Design review of the part built by this model. Coordinates are the model's own, in mm. A direction names the side the tool comes from. Give positions to 0.01 mm unless a question says otherwise; leave off trailing zeros. Loops run counter-clockwise (first coordinate to the right, second up) from the corner with the lowest first, then second, coordinate; pieces in that order, holes last. Notation, with made-up numbers: (11.25, 3) -> (31.25, 3) arc R25 ccw to (31.25, 30) -> close; hole circle Ø1 at (-8, 18.25). An arc over 180 degrees is marked (long way). Answer in a Markdown table with one row per item. Add a question column.
(1) Consider section D-D on y = 18. Write out the cut boundary in (x, z).
(2) For faces 1 (the cylindrical face through (17.923, -1.509, 1.726)), 2 (the flat face through (-48, 8.388, 2)), 3 (the flat face through (-38.16, -9.16, 1.73)), list the 3-axis set-ups (+Z, -Z, +X, -X, +Y, -Y) from which the entire face can be reached by the end or side of a thin tool; tool diameter is ignored.
(3) Consider section B-B on y = -14. Write out the cut boundary in (x, z).
(4) Consider section C-C on x = -63. Write out the cut boundary in (y, z), then the cut area to 3 significant figures.
(5) For pin 1 (1 mm diameter, centred on x = -53, z = 2, fed in from +Y); pin 2 (0.6 mm diameter, centred on y = 5, z = 3, fed in from -X); pin 3 (6 mm diameter, centred on x = 3, y = 2, fed in from -Z); pin 4 (4.5 mm diameter, centred on x = 14.28, y = 0, fed in from -Z), all flat-tipped, find the tip position at first contact; note any pin that passes through.
(6) Draft analysis for pull direction X (two halves, no side actions). For faces 4 (the flat face through (-25, -6.946, 2)), 5 (the flat face through (-11, 0, 3.5)), 6 (the flat face through (-84.457, -3.059, 1.726)), state which applies: +X half, -X half, draft (parallel to the pull), parting line (faces both ways), or undercut.
(7) Consider section A-A on z = 0.8. Write out the cut boundary in (x, y).
(8) For line 1 (X direction, y = -3.5, z = 1.6); line 2 (X direction, y = -3, z = 0.55); line 3 (Y direction, x = 12, z = 0.75), list the stretches that pass through material, from the lowest coordinate up.
from build123d import *

# Parameters (mm, degrees)
F0_R     = 3.93993
F1_DEPTH = 3.5
F4_DEPTH = 150


with BuildPart() as f1:
    # F0 (on Top) → F1 (new body)
    with BuildSketch(Plane.XY):
        with BuildLine():
            Line((-30.424483, -6.945617), (-19.31924, -6.945617))
            ThreePointArc((-19.31924, -6.945617), (20.515116, -0.777576), (-18.738052, 8.388087))
            Line((-18.738052, 8.388087), (-78.088284, 8.388087))
            Line((-78.088284, 8.388087), (-90.650834, 0.721235))
            Line((-90.650834, 0.721235), (-78.088284, -6.945617))
            Line((-78.088284, -6.945617), (-69.405347, -3.804978))
            Line((-69.405347, -3.804978), (-65.710478, -9.716768))
            Line((-65.710478, -9.716768), (-58.505483, -3.250748))
            Line((-58.505483, -3.250748), (-51.40605, -11.161547))
            Line((-51.40605, -11.161547), (-48.159853, -4.728695))
            Line((-48.159853, -4.728695), (-42.802293, -15.259069))
            Line((-42.802293, -15.259069), (-33.380378, -2.881262))
            Line((-33.380378, -2.881262), (-30.424483, -6.945617))
        make_face()
        with Locations((14.283421, 0)):
            Circle(F0_R, mode=Mode.SUBTRACT)
    extrude(amount=F1_DEPTH)

    # F3 (on offset) → F4 (cut)
    with BuildSketch(Plane.YZ.offset(-10)):
        Polygon((5.187124, 2.278307), (6.987329, 6.371124), (2.650907, 7.108018), align=None)
        Polygon((-2.074363, 2.495993), (-0.437801, 6.506958), (-4.136456, 7.135476), align=None)
    extrude(amount=-F4_DEPTH, mode=Mode.SUBTRACT)


solid = f1.part
Values follow:
| question | item | result |
|---|---|---|
| 1 | outline | (-9.87, 0) -> (9.87, 0) -> (9.87, 3.5) -> (-9.87, 3.5) -> close |
| 2 | face 1 | +Z, -Z |
| 2 | face 2 | +Z, -Z, -X, +Y |
| 2 | face 3 | +Z, -Z, -Y |
| 3 | outline | (-43.44, 0) -> (-41.84, 0) -> (-41.84, 3.5) -> (-43.44, 3.5) -> close; (-15.02, 0) -> (15.02, 0) -> (15.02, 3.5) -> (-15.02, 3.5) -> close |
| 4 | outline | (-7.28, 0) -> (8.39, 0) -> (8.39, 3.5) -> (5.72, 3.5) -> (5.19, 2.28) -> (4.55, 3.5) -> (-1.66, 3.5) -> (-2.07, 2.5) -> (-2.52, 3.5) -> (-7.28, 3.5) -> close |
| 4 | area | 53.7 mm2 |
| 5 | pin 1 | y = 8.39 |
| 5 | pin 2 | x = -84.13 |
| 5 | pin 3 | z = 0 |
| 5 | pin 4 | through |
| 6 | face 4 | undercut |
| 6 | face 5 | draft |
| 6 | face 6 | -X half |
| 7 | outline | (-90.65, 0.72) -> (-78.09, -6.95) -> (-69.41, -3.8) -> (-65.71, -9.72) -> (-58.51, -3.25) -> (-51.41, -11.16) -> (-48.16, -4.73) -> (-42.8, -15.26) -> (-33.38, -2.88) -> (-30.42, -6.95) -> (-19.32, -6.95) arc R20.53 ccw (long way) to (-18.74, 8.39) -> (-78.09, 8.39) -> close; hole circle Ø7.88 at (14.28, 0) |
| 8 | line 1 | -83.73 to -58.78, -58.28 to -33.85, -32.93 to 12.47, 16.09 to 20.23 |
| 8 | line 2 | -84.55 to -33.47, -33.29 to 11.73, 16.84 to 20.31 |
| 8 | line 3 | -16.66 to -3.21, 3.21 to 16.66 |
